Geometry: final body of the model. Coordinates: model frame, mm. Face numbers are marked on the shaded views. A direction names the side the tool comes from. Coordinates: 2 decimals unless noted, no trailing zeros. Write each loop counter-clockwise with the first axis right and the second up, starting at its lowest first coordinate (ties: lowest second). Pieces come first, ordered by that corner, then holes. Notation, with made-up numbers: (53.5, -3) - (93.5, -3) arc R14 cw to (93.5, 5) - close; hole circle Ø10 at (85, -37.5). An arc over 180 degrees is marked (long way). Answer as a JSON object with one key per item and string values. Group by question number.
Item 1: Section C-C on z = 1.8. Return loops of the section in (x, y) (3 decimals), and give its area (3 significant figures).
Item 2: Mould query, pull axis X, two halves, no side actions, for the marked faces 1, 2 and 3. Classes: pulls with the +X half, pulls with the -X half, needs draft (parallel to the pull), parting line crosses it, or undercut.
Item 3: Section B-B on y = 0. Return loops of the section in (x, z), and give its area (3 significant figures).
Item 4: Line query: line 1 along Y through (x, z) = (-21, 2.1); line 2 along Y through (x, z) = (13.5, 2.1); line 3 along X through (y, z) = (0.5, 3.2). Output: solid intervals per line, ascending. Write a range as from..to.
Item 5: Section A-A on x = 0. Return loops of the section in (y, z) (3 decimals), and give its area (3 significant figures).
Item 6: Section D-D on x = -20. Return loops of the section in (y, z).
Item 7: First-contact query: pin 1 Ø1.1 at (x, z) = (-2, 2) entering from -Y; pin 2 Ø3 at (x, y) = (0, -7.9) entering from +Z; pin 3 Ø4 at (x, y) = (-1, -7) entering from +Z; pin 4 Ø2 at (y, z) = (-4.5, 1) entering from -X. Flat tips, straight axial feed; report the tip coordinate or a pass-through.
Item 8: Set-up query: the marked faces 4 and 5. Return all of +Z, -Z, +X, -X, +Y, -Y with unobstructed straight access to the full face (end or side cutting, diameter ignored); none if empty.
Autodesk Inventor part; units mm, degrees
ref_plane "YZ Plane" through (0, 0, 0) normal (1, 0, 0) x (0, 1, 0)
ref_plane "XZ Plane" through (0, 0, 0) normal (0, 1, 0) x (-1, 0, 0)
ref_plane "XY Plane" through (0, 0, 0) normal (0, 0, 1) x (1, 0, 0)
sketch "Sketch1" plane through (0, 0, 0) normal (0, 0, 1) x (1, 0, 0)
  circle A0 centre (0, 0) radius 25.5
  dimension "d0" = 51
extrude "Extrusion1" add sketch "Sketch1" along normal blind 3.6
sketch "Sketch2" plane through (0, 0, 3.6) normal (0, 0, 1) x (1, 0, 0)
  line L0 (17.5, 0) -> (-17.5, 0) construction
  line L1 (17.5, 6.15) -> (-17.5, 6.15)
  line L2 (-17.5, -6.15) -> (17.5, -6.15)
  arc A0 (17.5, -6.15) -> (17.5, 6.15) centre (17.5, 0) ccw
  arc A1 (-17.5, 6.15) -> (-17.5, -6.15) centre (-17.5, 0) ccw
  point P0 (0, 0)
  dimension "d3" = 17.5
  dimension "d4" = 12.3
extrude "Extrusion2" cut sketch "Sketch2" against normal blind 3.6
sketch "Sketch3" plane through (0, 0, 3.6) normal (0, 0, 1) x (1, 0, 0)
  line L0 (-2.6, 9.8) -> (2.6, 9.8)
  line L1 (2.6, 9.8) -> (2.6, 6)
  line L2 (2.6, 6) -> (-2.6, 6)
  line L3 (-2.6, 6) -> (-2.6, 9.8)
  line L4 (-2.6, 9.8) -> (2.6, 6) construction
  line L5 (2.6, 9.8) -> (-2.6, 6) construction
  line L6 (-35.7, 0) -> (35.7, 0)
  line L7 (-35.7, 0) -> (35.7, 0)
  line L8 (-2.6, -9.8) -> (2.6, -9.8)
  line L9 (2.6, -9.8) -> (2.6, -6)
  line L10 (2.6, -6) -> (-2.6, -6)
  line L11 (-2.6, -6) -> (-2.6, -9.8)
  line L12 (-2.6, -9.8) -> (2.6, -6) construction
  line L13 (2.6, -9.8) -> (-2.6, -6) construction
  circle A0 centre (0, -7.9) radius 1.625
  circle A1 centre (0, 7.9) radius 1.625
  point P0 (0, 0)
  dimension "d7" = 5.2
  dimension "d8" = 3.8
  dimension "d9" = 6
  dimension "d10" = 6
  dimension "d13" = 0
  dimension "d14" = 3.25
  dimension "d15" = 3.25
extrude "Extrusion3" cut sketch "Sketch3" against normal blind 10 contours A0 | A1
properties part number "1"
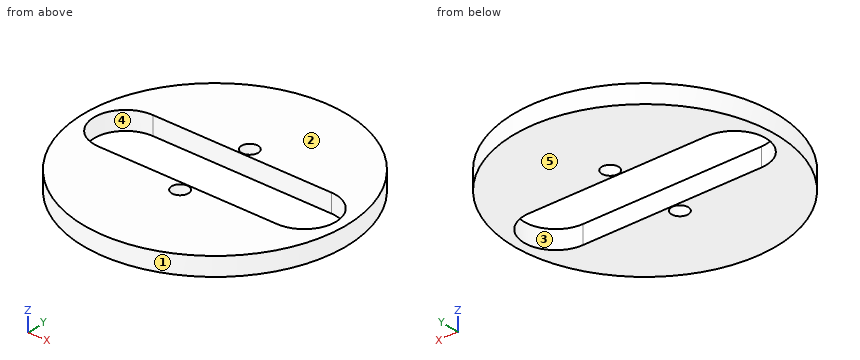
Checks:
{
 "1": {"outline": "circle Ø51 at (0, 0); hole (-17.5, -6.15) - (17.5, -6.15) arc R6.15 ccw to (17.5, 6.15) - (-17.5, 6.15) arc R6.15 ccw to start; hole circle Ø3.25 at (0, -7.9); hole circle Ø3.25 at (0, 7.9)", "area": "1,480 mm^2"},
 "2": {"face 1": "parting line crosses it", "face 2": "needs draft", "face 3": "undercut"},
 "3": {"outline": "(-25.5, 0) - (-23.65, 0) - (-23.65, 3.6) - (-25.5, 3.6) - close; (23.65, 0) - (25.5, 0) - (25.5, 3.6) - (23.65, 3.6) - close", "area": "13.3 mm^2"},
 "4": {"line 1": "-14.47..-5.06, 5.06..14.47", "line 2": "-21.63..-6.15, 6.15..21.63", "line 3": "-25.5..-23.63, 23.63..25.5"},
 "5": {"outline": "(-25.5, 0) - (-9.525, 0) - (-9.525, 3.6) - (-25.5, 3.6) - close; (-6.275, 0) - (-6.15, 0) - (-6.15, 3.6) - (-6.275, 3.6) - close; (6.15, 0) - (6.275, 0) - (6.275, 3.6) - (6.15, 3.6) - close; (9.525, 0) - (25.5, 0) - (25.5, 3.6) - (9.525, 3.6) - close", "area": "116 mm^2"},
 "6": {"outline": "(-15.82, 0) - (-5.62, 0) - (-5.62, 3.6) - (-15.82, 3.6) - close; (5.62, 0) - (15.82, 0) - (15.82, 3.6) - (5.62, 3.6) - close"},
 "7": {"pin 1": "y = -25.46", "pin 2": "through", "pin 3": "z = 3.6", "pin 4": "x = -25.26"},
 "8": {"face 4": "+Z, -Z", "face 5": "-Z, +X, -X, +Y, -Y"}
}
